Autodesk Fusion 360 part; units mm, degrees
sketch "Body" plane through (0, 0, 0) normal (0, 1, 0) x (1, 0, 0)
  line L0 (-22.5, -22.5) -> (22.5, -22.5)
  line L1 (22.5, -22.5) -> (22.5, 22.5)
  line L2 (22.5, 22.5) -> (-22.5, 22.5)
  line L3 (-22.5, 22.5) -> (-22.5, -22.5)
  line L4 (-22.5, -22.5) -> (22.5, 22.5) construction
  line L5 (22.5, -22.5) -> (-22.5, 22.5) construction
  line L6 (22.4, 22.4) -> (-22.4, 22.4)
  line L7 (-22.4, 22.4) -> (-22.4, -22.4)
  line L8 (-22.4, -22.4) -> (22.4, -22.4)
  line L9 (22.4, -22.4) -> (22.4, 22.4)
  line L10 (-21.2, 21.2) -> (-21.2, -21.2)
  line L11 (-21.2, -21.2) -> (21.2, -21.2)
  line L12 (21.2, -21.2) -> (21.2, 21.2)
  line L13 (21.2, 21.2) -> (-21.2, 21.2)
  line L14 (-22.5, -22.5) -> (-15.7, -22.5) construction
  line L15 (-15.7, -22.5) -> (-15.7, -22.4) construction
  line L16 (-15.7, -22.4) -> (-22.5, -22.4) construction
  line L17 (-22.5, -22.4) -> (-22.5, -22.5) construction
  line L18 (-22.5, -22.5) -> (-22.4, -22.5) construction
  line L19 (-22.4, -22.5) -> (-22.4, -14.4) construction
  line L20 (-22.4, -14.4) -> (-22.5, -14.4) construction
  line L21 (-22.5, -14.4) -> (-22.5, -22.5) construction
  line L22 (-22.4, -14.4) -> (-23.9, -14.4)
  line L23 (-23.9, -14.4) -> (-23.9, -15.6)
  line L24 (-23.9, -15.6) -> (-22.4, -15.6)
  line L25 (-22.4, -15.6) -> (-22.4, -14.4)
  line L26 (-15.7, -22.4) -> (-14.3, -22.4)
  line L27 (-14.3, -22.4) -> (-14.3, -20.9)
  line L28 (-14.3, -20.9) -> (-15.7, -20.9)
  line L29 (-15.7, -20.9) -> (-15.7, -22.4)
  line L30 (-13.1, -22.4) -> (-13.1, -19.7)
  line L31 (-13.1, -19.7) -> (-16.9, -19.7)
  line L32 (-16.9, -19.7) -> (-16.9, -22.4)
  line L33 (0, -22.5) -> (0, -28) construction
  line L34 (-22.5, 0) -> (-38.981, 0) construction
  line L35 (-22.5, 22.5) -> (-14.4, 22.5) construction
  line L36 (-14.4, 22.5) -> (-14.4, 22.4) construction
  line L37 (-14.4, 22.4) -> (-22.5, 22.4) construction
  line L38 (-22.5, 22.4) -> (-22.5, 22.5) construction
  line L39 (22.5, -22.5) -> (22.4, -22.5) construction
  line L40 (22.4, -22.5) -> (22.4, -15.7) construction
  line L41 (22.4, -15.7) -> (22.5, -15.7) construction
  line L42 (22.5, -15.7) -> (22.5, -22.5) construction
  line L43 (-14.4, 22.4) -> (-15.6, 22.4)
  line L44 (-15.6, 22.4) -> (-15.6, 23.9)
  line L45 (-15.6, 23.9) -> (-14.4, 23.9)
  line L46 (-14.4, 23.9) -> (-14.4, 22.4)
  line L47 (22.4, 16.2) -> (-22.4, 16.2)
  line L48 (22.4, -15.7) -> (20.9, -15.7)
  line L49 (20.9, -15.7) -> (20.9, -14.3)
  line L50 (20.9, -14.3) -> (22.4, -14.3)
  line L51 (22.4, -14.3) -> (22.4, -15.7)
  line L52 (22.4, -16.9) -> (19.7, -16.9)
  line L53 (19.7, -16.9) -> (19.7, -13.1)
  line L54 (19.7, -13.1) -> (22.4, -13.1)
  dimension "d39" = 45
  dimension "d40" = 45
  dimension "d43" = 6.8
  dimension "d44" = 0.1
  dimension "d45" = 0.1
  dimension "d46" = 8.1
  dimension "d47" = 1.5
  dimension "d48" = 1.2
  dimension "d49" = 1.4
  dimension "d50" = 1.5
  dimension "d51" = 1.2
  dimension "d66" = 8.1
  dimension "d67" = 0.1
  dimension "d70" = 0.1
  dimension "d71" = 6.8
  dimension "d81" = 1.2
  dimension "d82" = 1.5
  dimension "d196" = 1.5
  dimension "d197" = 1.4
extrude "Extrude1" add sketch "Body" along normal blind 110 contours L7 L8 L10 L11 L25 L32 L47 | L6 L7 L9 L10 L12 L13 L43 L47 | L8 L11 L29 L32 | L8 L11 L26 L27 L29 | L9 L12 L47 L54 | L8 L11 L27 L30 | L9 L12 L50 L54 | L8 L9 L11 L12 L30 L52 | L9 L12 L48 L50 L51 | L9 L12 L48 L52 makes body 1
ref_plane "WorkPlane3" through (0, 55, 0) normal (0, 1, 0) x (0, 0, 1)
sketch "Floor" plane through (0, 55, 0) normal (0, 1, 0) x (1, 0, 0)
  line L0 (-22.5, -22.5) -> (22.5, -22.5)
  line L1 (22.5, -22.5) -> (22.5, 22.5)
  line L2 (22.5, 22.5) -> (-22.5, 22.5)
  line L3 (-22.5, 22.5) -> (-22.5, -22.5)
  line L4 (-22.5, -22.5) -> (22.5, 22.5) construction
  line L5 (22.5, -22.5) -> (-22.5, 22.5) construction
  line L6 (-22.4, 22.4) -> (-22.4, -22.4)
  line L7 (-22.4, -22.4) -> (22.4, -22.4)
  line L8 (22.4, -22.4) -> (22.4, 22.4)
  line L9 (22.4, 22.4) -> (-22.4, 22.4)
  line L10 (-21.3, 21.3) -> (-21.3, -21.3)
  line L11 (-21.3, -21.3) -> (21.3, -21.3)
  line L12 (21.3, -21.3) -> (21.3, 21.3)
  line L13 (21.3, 21.3) -> (-21.3, 21.3)
  line L14 (0, 21.3) -> (-20.6, 21.3) construction
  line L15 (-20.6, 21.3) -> (-20.6, 21.1) construction
  line L16 (-20.6, 21.1) -> (0, 21.1) construction
  line L17 (0, 21.1) -> (0, 21.3) construction
  line L18 (0, 21.3) -> (19.1, 21.3) construction
  line L19 (19.1, 21.3) -> (19.1, 21.1) construction
  line L20 (19.1, 21.1) -> (0, 21.1) construction
  line L21 (0, 21.1) -> (0, 21.3) construction
  line L22 (-20.6, 21.1) -> (-21.7, 21.1)
  line L23 (-21.7, 21.1) -> (-21.7, 20.1)
  line L24 (-21.7, 20.1) -> (-20.6, 20.1)
  line L25 (-20.6, 20.1) -> (-20.6, 21.1)
  line L26 (-21.7, 20.1) -> (-20.6, 21.1)
  line L27 (19.1, 21.1) -> (20.2, 21.1)
  line L28 (20.2, 21.1) -> (20.2, 20.1)
  line L29 (20.2, 20.1) -> (19.1, 20.1)
  line L30 (19.1, 20.1) -> (19.1, 21.1)
  line L31 (19.1, 21.1) -> (20.2, 20.1)
  dimension "d219" = 45
  dimension "d220" = 45
  dimension "d243" = 20.6
  dimension "d244" = 0.2
  dimension "d245" = 19.1
  dimension "d246" = 0.2
  dimension "d247" = 1.1
  dimension "d248" = 1
  dimension "d249" = 1.1
  dimension "d250" = 1
extrude "Extrude19" add sketch "Floor" along normal blind 1 from surface at -55 contours L10 L11 L12 L13 L22 L24 L25 | L10 L22 L26 | L10 L24 L25 L26 | L29 L30 L31 | L27 L28 L31 bodies 1
extrude "Extrude3" add sketch "Body" along normal blind 110 contours L8 L11 L29 L32 | L11 L27 L28 L29 L30 L31 L32 | L8 L11 L27 L30 bodies 1
extrude "Extrude4" cut sketch "Body" along normal blind 110 contours L8 L11 L26 L27 L29 | L11 L27 L28 L29 bodies 1
extrude "Extrude8" add sketch "Body" along normal blind 110 contours L2 L6 L43 L44 L46 | L2 L44 L45 L46 bodies 1
extrude "Extrude5" add sketch "Body" along normal blind 110 contours L3 L22 L23 L24 | L3 L7 L22 L24 L25 bodies 1
extrude "Extrude6" add sketch "Body" along normal blind 110 contours L9 L12 L50 L54 | L12 L48 L49 L50 L52 L53 L54 | L9 L12 L48 L52 bodies 1
extrude "Extrude7" cut sketch "Body" along normal blind 110 contours L9 L12 L48 L50 L51 | L12 L48 L49 L50 bodies 1
pattern_linear "R-Pattern1" count 3 spacing 15 along (1, 0, 0) of "Extrude3", "Extrude4", "Extrude8"
pattern_linear "R-Pattern2" count 3 spacing 15 along (0, 0, -1) of "Extrude5", "Extrude7", "Extrude6"
extrude "Extrude15" add sketch "Body" along normal blind 5 from surface at 110 contours L6 L7 L9 L10 L12 L13 L43 L47 bodies 1
chamfer "Chamfer1" distance 5 angle 45 2 edges at (21.8, 115, -16.2) (-21.8, 115, -16.2) on bodies 1
sketch "Pull Tab Hole" plane through (0, 0, 0) normal (0, 0, 1) x (1, 0, 0)
  line L0 (0, 0) -> (0, 110) construction
  line L1 (0, 110) -> (0, 112.5) construction
  line L2 (3.726, 113.8) -> (-3.726, 113.8)
  line L3 (-5, 112.526) -> (-5, 112.474)
  line L4 (-3.726, 111.2) -> (3.726, 111.2)
  line L5 (5, 112.474) -> (5, 112.526)
  line L6 (5, 113.8) -> (-5, 111.2) construction
  line L7 (-5, 113.8) -> (5, 111.2) construction
  arc A0 (-5, 112.474) -> (-3.726, 111.2) centre (-3.726, 112.474) ccw
  arc A1 (-3.726, 113.8) -> (-5, 112.526) centre (-3.726, 112.526) ccw
  arc A2 (5, 112.526) -> (3.726, 113.8) centre (3.726, 112.526) ccw
  arc A3 (3.726, 111.2) -> (5, 112.474) centre (3.726, 112.474) ccw
  point P0 (0, 112.5)
  dimension "d180" = 110
  dimension "d181" = 2.5
  dimension "d182" = 10
  dimension "d183" = 2.6
  dimension "d184" = 1.274
extrude "Extrude16" cut sketch "Pull Tab Hole" against normal blind 45 bodies 1
copy_body "Body->Comp3" bodies 1 removing the originals makes body 2 in component "Body"
component "Body" placed x (1, 0, 0) y (0, 1, 0) z (0, 0, 1) at (0, 0, 0)
equation "GRID_SPACING = 15 mm"
equation "WALL_THICK = 1.2 mm"
equation "WALL_BUMP = 1.5 mm"
equation "CLEAR = 0.1 mm"
equation "OVERALL_HT = 110 mm"
equation "FLOOR_THICK = 1 mm"
equation "d31 = OVERALL_HT"
equation "d35 = OVERALL_HT"
equation "d37 = OVERALL_HT"
equation "d39 = LENGTH_MODULE_NUMBER * GRID_SPACING"
equation "d40 = WIDTH_MODULE_NUMBER * GRID_SPACING"
equation "d43 = GRID_SPACING / 2 - WALL_THICK / 2 - CLEAR"
equation "d44 = CLEAR"
equation "d45 = CLEAR"
equation "d46 = GRID_SPACING / 2 + WALL_THICK / 2"
equation "d47 = WALL_BUMP"
equation "d48 = WALL_THICK"
equation "d49 = WALL_THICK + CLEAR * 2"
equation "d50 = WALL_BUMP"
equation "d51 = WALL_THICK"
equation "d54 = GRID_SPACING"
equation "d56 = OVERALL_HT"
equation "d60 = GRID_SPACING"
equation "d66 = GRID_SPACING / 2 + WALL_THICK / 2"
equation "d67 = CLEAR"
equation "d70 = CLEAR"
equation "d71 = GRID_SPACING / 2 - WALL_THICK / 2 - CLEAR"
equation "d75 = OVERALL_HT"
equation "d77 = OVERALL_HT"
equation "d79 = OVERALL_HT"
equation "d81 = WALL_THICK"
equation "d82 = WALL_BUMP"
equation "LID_THICK = 3 mm"
equation "LID_TOP_OFFSET = 1 mm"
equation "LID_LOCK_LENGTH = 8 mm"
equation "LID_PULL_WIDTH = 8 mm"
equation "LID_PULL_HT = 1 mm"
equation "LID_PULL_FRONT_OFFSET = 3 mm"
equation "PULL_TAB_WIDTH = PULL_TAB_HT + WALL_THICK"
equation "d173 = OVERALL_HT"
equation "d174 = PULL_TAB_HT"
equation "PULL_TAB_HT = 5 mm"
equation "d179 = PULL_TAB_HT"
equation "d180 = OVERALL_HT"
equation "d181 = PULL_TAB_HT / 2"
equation "d182 = PULL_HOLE_LENGTH"
equation "d183 = PULL_TAB_HT - WALL_THICK * 2"
equation "d184 = ( PULL_TAB_HT - WALL_THICK * 2 ) * 0.49"
equation "PULL_HOLE_LENGTH = 10 mm"
equation "d196 = WALL_BUMP"
equation "d197 = WALL_THICK + CLEAR * 2"
equation "d200 = OVERALL_HT / 2"
equation "d219 = LENGTH_MODULE_NUMBER * GRID_SPACING"
equation "d220 = WIDTH_MODULE_NUMBER * GRID_SPACING"
equation "d223 = FLOOR_THICK"
equation "LID_CLEAR = 0.1 mm"
equation "CHAMFER_LENGTH = 0.5 mm"
equation "CHAMFER_WIDTH = 1 mm"
equation "d243 = Linear Dimension-6"
equation "d244 = LID_CLEAR + CLEAR"
equation "d245 = Linear Dimension-8"
equation "d246 = LID_CLEAR + CLEAR"
equation "d247 = WALL_THICK / 2 + CHAMFER_LENGTH"
equation "d248 = CHAMFER_WIDTH"
equation "d249 = WALL_THICK / 2 + CHAMFER_LENGTH"
equation "d250 = CHAMFER_WIDTH"
equation "d253 = -OVERALL_HT / 2"
equation "LID_LOCK_OFFSET = 0.1 mm"
The listing builds one solid part. Answer for the finished solid, in the listing's coordinates (mm). A direction names the side the tool comes from. Round coordinates to 2 decimals unless told otherwise and drop trailing zeros. Loops run counter-clockwise (first coordinate to the right, second up) from the corner with the lowest first, then second, coordinate; pieces in that order, holes last.
Q1. Find the intervals of material crossed by line 1 (Z direction, x = 14.5, y = 86); line 2 (X direction, y = 81.5, z = -9.5); line 3 (Z direction, x = -14, y = 80.5), in increasing order.
Q2. Given pin 1 Ø3 at (x, z) = (8.5, 10) entering from +Y; pin 2 Ø1.2 at (x, y) = (20.5, 32) entering from -Z; pin 3 Ø0.6 at (x, z) = (-15, -23.5) entering from +Y, each flat-ended and moving along its own axis, determine where each tip first touches the part or whether it passes through.
Q3. Which of the six approach directions +Z, -Z, +X, -X, +Y, -Y give full straight-line access (tool end or side, diameter ignored) to faces 4 (the face through (-8, 55, 21.2)), 5 (the face through (-19, 54, 22.4))?
Q4. For a pull along X with two mould halves and no side action, classify faces 1 (the face through (22.4, 54, -7)), 2 (the face through (-19, 55, 21.2)), 3 (the face through (-8, 54, 22.4)) as released by +X, released by -X, zero draft, split by the parting line, or undercut.
Q5. Section B-B, the plane x = -8.5 is taken. Determine the outline of the cut face in (y, z), then the cut area to 3 significant figures.
Q6. Section A-A, the plane z = 18.5 is taken. Determine the outline of the cut face in (x, y), then the cut area to 3 significant figures.
Completed:
1. line 1: z = -23.9 to -21.2, 19.7 to 20.9
1. line 2: x = -22.4 to -21.2, 21.2 to 22.4
1. line 3: z = -22.4 to -21.2, 19.7 to 22.4
2. pin 1: stops at y = 1
2. pin 2: stops at z = -22.4
2. pin 3: stops at y = 110
3. face 4: +Y
3. face 5: +Z, +X, -X, +Y, -Y
4. face 1: released by +X
4. face 2: undercut
4. face 3: zero draft
5. outline: (0, -22.4) - (115, -22.4) - (115, -21.2) - (1, -21.2) - (1, 21.2) - (110, 21.2) - (110, 22.4) - (0, 22.4) - close
5. area: 312 mm2
6. outline: (-22.4, 0) - (22.4, 0) - (22.4, 110) - (21.2, 110) - (21.2, 1) - (-21.2, 1) - (-21.2, 110) - (-22.4, 110) - close
6. area: 306 mm2
